```python
from build123d import *

# Parameters (mm, degrees)
EXTRUDE1_DEPTH     = 28.067
CUT_EXTRUDE1_DEPTH = 32.75
SKETCH3_R          = 5.54355
CUT_EXTRUDE2_DEPTH = 32.75
FILLET1_R          = 1.524
FILLET2_R          = 0.508
FILLET3_R          = 1.524


with BuildPart() as part:
    # Sketch1 → Extrude1 (new body)
    with BuildSketch(Plane(origin=(0, 0, 0), x_dir=(1, 0, 0), z_dir=(0, 1, 0))):
        Polygon((-9.525, 107.95), (9.525, 107.95), (9.525, 45.212), (15.875, 14.224508), (15.875, -14.224508), (9.525, -45.212), (9.525, -107.95), (-9.525, -107.95), (-9.525, -45.212), (-15.875, -14.224508), (-15.875, 14.224508), (-9.525, 45.212), align=None)
        with BuildLine():
            Line((-6.7818, 8.8265), (-6.7818, -8.8265))
            ThreePointArc((-6.7818, -8.8265), (0, -15.6083), (6.7818, -8.8265))
            Line((6.7818, -8.8265), (6.7818, 8.8265))
            ThreePointArc((6.7818, 8.8265), (0, 15.6083), (-6.7818, 8.8265))
        make_face(mode=Mode.SUBTRACT)
    extrude(amount=EXTRUDE1_DEPTH)

    # Sketch2 → Cut-Extrude1 (cut, through all)
    with BuildSketch(Plane(origin=(15.875, 0, 0), x_dir=(0, 0, -1), z_dir=(1, 0, 0))):
        Polygon((107.95, 28.067), (18.5674, 28.067), (46.074990269, 15.24), (107.95, 15.24), align=None)
        Polygon((-107.95, 15.24), (-107.95, 28.067), (-18.5674, 28.067), (-46.074990269, 15.24), align=None)
    extrude(amount=-CUT_EXTRUDE1_DEPTH, mode=Mode.SUBTRACT)

    # Sketch3 → Cut-Extrude2 (cut, through all)
    with BuildSketch(Plane(origin=(15.875, 0, 0), x_dir=(0, 0, -1), z_dir=(1, 0, 0))):
        with Locations((0, 13.9446)):
            Circle(SKETCH3_R)
    extrude(amount=-CUT_EXTRUDE2_DEPTH, mode=Mode.SUBTRACT)

    # Fillet1
    fillet1_edges = [part.edges().sort_by_distance(p)[0] for p in [
        (-9.525, 7.62, -107.95),
        (9.525, 7.62, -107.95),
        (9.525, 7.62, 107.95),
        (-9.525, 7.62, 107.95),
    ]]
    fillet(fillet1_edges, radius=FILLET1_R)

    # Fillet2
    fillet2_edges = [part.edges().sort_by_distance(p)[0] for p in [
        (-9.525, 0, -75.819),
        (9.525, 0, 75.819),
        (0, 0, 107.95),
        (0, 0, -107.95),
        (-9.078630735, 0, 107.503630735),
        (12.7, 0, -29.718254),
        (9.078630735, 0, 107.503630735),
        (9.078630735, 0, -107.503630735),
        (-9.078630735, 0, -107.503630735),
        (15.875, 0, 0),
        (12.7, 0, 29.718254),
        (-9.525, 0, 75.819),
        (-12.7, 0, 29.718254),
        (-15.875, 0, 0),
        (-12.7, 0, -29.718254),
        (9.525, 0, -75.819),
    ]]
    fillet(fillet2_edges, radius=FILLET2_R)

    # Fillet3
    fillet3_edges = [part.edges().sort_by_distance(p)[0] for p in [
        (0, 15.24, -107.95),
        (9.525, 15.24, -76.250495135),
        (9.078630735, 15.24, -107.503630735),
        (-9.078630735, 15.24, -107.503630735),
        (0, 15.24, 107.95),
        (-9.525, 15.24, 76.250495135),
        (-9.078630735, 15.24, 107.503630735),
        (9.078630735, 15.24, 107.503630735),
        (-15.875, 28.067, 0),
        (-15.430024263, 28.067, 16.395954),
        (15.875, 28.067, 0),
        (15.430024263, 28.067, -16.395954),
        (12.255024263, 21.854709486, -31.8897),
        (-15.430024263, 28.067, -16.395954),
        (-9.525, 15.24, -76.250495135),
        (-12.255024263, 21.854709486, -31.8897),
        (-9.525, 15.441209486, -45.643495135),
        (9.525, 15.441209486, -45.643495135),
        (15.430024263, 28.067, 16.395954),
        (12.255024263, 21.854709486, 31.8897),
        (9.525, 15.24, 76.250495135),
        (-9.525, 15.441209486, 45.643495135),
        (-12.255024263, 21.854709486, 31.8897),
        (9.525, 15.441209486, 45.643495135),
    ]]
    fillet(fillet3_edges, radius=FILLET3_R)


solid = part.part
```
Input: part model. Units: mm. Frame: model coordinates. A direction names the side the tool comes from. Coordinates: 2 decimals unless noted, no trailing zeros. Write each loop counter-clockwise with the first axis right and the second up, starting at its lowest first coordinate (ties: lowest second). Pieces come first, ordered by that corner, then holes. Notation, with made-up numbers: M 73,87.5 L 131,87.5 A23 cw 131,117.5 Z; hole C 44.25,78 d11. An arc over 180 degrees is marked long. Use one line per item in the form item = value.
Q1. Set-up query: faces 1 (the face through (-6.782, 14, 6)), 2 (the face through (9.525, 7, -76)), 3 (the face through (0, 15.24, 76)). Return all of +Z, -Z, +X, -X, +Y, -Y with unobstructed straight access to the full face (end or side cutting, diameter ignored); none if empty.
Answer below:
face_1 = +Y, -Y
face_2 = -Z, +X, +Y, -Y
face_3 = +Z, +X, -X, +Y
Q2. Section A-A (x = 0). Return loops of the section in (y, z) (3 decimals).
Answer below:
outline = M 0,-107.442 A0.508 ccw 0.508,-107.95 L 13.716,-107.95 A1.524 ccw 15.24,-106.426 L 15.24,-46.075 L 28.067,-18.567 L 28.067,-15.608 L 0,-15.608 Z; M 0,15.608 L 28.067,15.608 L 28.067,18.567 L 15.24,46.075 L 15.24,106.426 A1.524 ccw 13.716,107.95 L 0.508,107.95 A0.508 ccw 0,107.442 Z
Q3. Section B-B (z = 0). Return loops of the section in (x, y) (3 decimals).
Answer below:
outline = M -15.875,0.508 A0.508 ccw -15.367,0 L -6.782,0 L -6.782,8.401 L -15.875,8.401 Z; M -15.875,19.488 L -6.782,19.488 L -6.782,28.067 L -14.351,28.067 A1.524 ccw -15.875,26.543 Z; M 6.782,0 L 15.367,0 A0.508 ccw 15.875,0.508 L 15.875,8.401 L 6.782,8.401 Z; M 6.782,19.488 L 15.875,19.488 L 15.875,26.543 A1.524 ccw 14.351,28.067 L 6.782,28.067 Z
Q4. Section D-D (z = 87.5). Return loops of the section in (x, y) (3 decimals).
Answer below:
outline = M -9.525,0.508 A0.508 ccw -9.017,0 L 9.017,0 A0.508 ccw 9.525,0.508 L 9.525,13.716 A1.524 ccw 8.001,15.24 L -8.001,15.24 A1.524 ccw -9.525,13.716 Z
Q5. Draft query along Z for faces 4 (the face through (-0.149, 13.837, 15.607)), 5 (the face through (12.59, 0.145, -29.496)), 6 (the face through (0, 15.24, -76)), 7 (the face through (12.501, 0.145, 29.93)). Return one class per face: released by +Z, released by -Z, zero draft, split by the parting line, or undercut.
Answer below:
face_4 = undercut
face_5 = released by -Z
face_6 = zero draft
face_7 = released by +Z
Q6. Material intervals for probe 1 along Y at (x, z) = (13, 0); probe 2 along X at (y, z) = (26.25, -9) (3 decimals); probe 3 along X at (y, z) = (11, 67) (3 decimals), sorted ascending. Write a range as from..to.
Answer below:
probe_1 = 0..8.4, 19.49..28.07
probe_2 = -15.875..-6.78, 6.78..15.875
probe_3 = -9.525..9.525
Q7. First-contact query: pin 1 (13 mm diameter, centred on x = 0, z = 88, fed in from +Y); pin 2 (4 mm diameter, centred on y = 9.5, z = -86, fed in from +X) (3 decimals); pin 3 (2 mm diameter, centred on x = 1, y = 23.5, fed in from +Z). Flat tips, straight axial feed; report the tip coordinate or a pass-through.
Answer below:
pin_1 = 15.24
pin_2 = 9.525
pin_3 = 30.51
